Build history of the part. All positions in model axes, mm. A direction names the side the tool comes from. Give positions to 0.01 mm unless a question says otherwise; leave off trailing zeros. Loops run counter-clockwise (first coordinate to the right, second up) from the corner with the lowest first, then second, coordinate; pieces in that order, holes last. Notation, with made-up numbers: (30, 53.5) -> (86, 53.5) arc R6 cw to (86, 63.5) -> close; hole circle Ø1 at (-28, 38). An arc over 180 degrees is marked (long way). One line per question, with ' | ' between items. Start each with the question number.
(1) Mould opens along X. For faces 1 (the face through (-48.22, 2.5, 0.48)), 2 (the face through (11.437, 12.629, -13.635)), 3 (the face through (-0.64, 2.5, 36.79)) say: pulls with the +X half, pulls with the -X half, needs draft (parallel to the pull), parting line crosses it, or undercut.
(2) Slice it at C-C, the plane y = 9. Write the cut outline in (x, z).
(3) Flat gauge pins, fed straight in: pin 1 Ø2 at (x, z) = (30, -6.5) entering from -Y; pin 2 Ø7.5 at (x, z) = (-20, 12.5) entering from -Y; pin 3 Ø17.5 at (y, z) = (41.91, 0) entering from -X. Where does each tip first touch, or does it go through?
(4) Slice it at B-B, the plane x = 4.5. Write the cut outline in (y, z).
(5) 3-axis set-ups, long thin cutter, end or side, ignore diameter. For faces 4 (the face through (48.224, 84.364, -0.373)), 5 (the face through (-1, 7.62, 0)): which of +Z, -Z, +X, -X, +Y, -Y reach the whole face in a straight line?
(6) Drill centre lines: L1, parallel to Z at x = 19, y = 10; L2, parallel to X at y = 12, z = -14.5; L3, parallel to Z at x = 40, y = 41.91. Where is each one in solid material? Low to high. Write a range as from..to.
(7) Slice it at A-A, the plane z = -13.97. Write the cut outline in (x, y), then the cut area to 3 significant figures.
(8) Slice it at D-D, the plane y = 70.5. Write the cut outline in (x, z), then the cut area to 3 significant figures.
```python
from build123d import *

# Parameters (mm, degrees)
F1_DEPTH = 50.8
F2_W     = 76.2
F2_H     = 53.34
F3_DEPTH = 7.62
F4_R     = 7.62
F5_DEPTH = 10.16
F6_R     = 7.62
F7_DEPTH = 19.05
F8_R     = 7.62
F9_DEPTH = 19.05
F10_SIZE = 5.08


with BuildPart() as f1:
    # F0 (on Right) → F1 (new body, symmetric)
    with BuildSketch(Plane.YZ):
        Polygon((41.91, 39.37), (0, 39.37), (0, 0), (0, -39.37), (41.91, -39.37), (86.868, -26.67), (86.868, 0), (86.868, 26.67), align=None)
    extrude(amount=F1_DEPTH, both=True)

    # F2 (on face) → F3 (cut)
    with BuildSketch(Plane.XZ):
        Rectangle(F2_W, F2_H)
    extrude(amount=-F3_DEPTH, mode=Mode.SUBTRACT)

    # F4 (on face) → F5 (cut)
    with BuildSketch(Plane.XZ.offset(-7.62)):
        with Locations((-19.05, 13.97)):
            Circle(F4_R)
        with Locations((19.05, 13.97)):
            Circle(F4_R)
        with Locations((-19.05, -13.97)):
            Circle(F4_R)
        with Locations((19.05, -13.97)):
            Circle(F4_R)
    extrude(amount=-F5_DEPTH, mode=Mode.SUBTRACT)

    # F6 (on face) → F7 (cut)
    with BuildSketch(Plane.YZ.offset(50.8)):
        with Locations((41.91, 0)):
            Circle(F6_R)
    extrude(amount=-F7_DEPTH, mode=Mode.SUBTRACT)

    # F8 (on face) → F9 (cut)
    with BuildSketch(Plane(origin=(-50.8, 0, 0), x_dir=(0, -1, 0), z_dir=(-1, 0, 0))):
        with Locations((-41.91, 0)):
            Circle(F8_R)
    extrude(amount=-F9_DEPTH, mode=Mode.SUBTRACT)

    # F10
    f10_edges = [f1.edges().sort_by_distance(p)[0] for p in [
        (50.8, 20.955, 39.37),
        (50.8, 64.389, 33.02),
        (50.8, 0, 0),
        (50.8, 86.868, 0),
        (50.8, 20.955, -39.37),
        (50.8, 64.389, -33.02),
        (50.8, 34.29, 0),
        (-50.8, 20.955, 39.37),
        (-50.8, 64.389, 33.02),
        (-50.8, 0, 0),
        (-50.8, 86.868, 0),
        (-50.8, 20.955, -39.37),
        (-50.8, 64.389, -33.02),
        (-50.8, 49.53, 0),
        (0, 0, 39.37),
        (0, 0, -39.37),
    ]]
    chamfer(f10_edges, length=F10_SIZE)


solid = f1.part
```
Final values:
1) face 1: pulls with the -X half | face 2: undercut | face 3: needs draft
2) outline: (-50.8, -34.29) -> (-45.72, -39.37) -> (45.72, -39.37) -> (50.8, -34.29) -> (50.8, 34.29) -> (45.72, 39.37) -> (-45.72, 39.37) -> (-50.8, 34.29) -> close; hole circle Ø15.24 at (-19.05, -13.97); hole circle Ø15.24 at (-19.05, 13.97); hole circle Ø15.24 at (19.05, -13.97); hole circle Ø15.24 at (19.05, 13.97)
3) pin 1: y = 7.62 | pin 2: y = 17.78 | pin 3: x = -46.85
4) outline: (0, -34.29) -> (5.08, -39.37) -> (41.91, -39.37) -> (86.87, -26.67) -> (86.87, 26.67) -> (41.91, 39.37) -> (5.08, 39.37) -> (0, 34.29) -> (0, 26.67) -> (7.62, 26.67) -> (7.62, -26.67) -> (0, -26.67) -> close
5) face 4: +Z, -Z, +X, +Y | face 5: -Y
6) L1: -39.37..-21.59, -6.35..6.35, 21.59..39.37 | L2: -50.8..-26.65, -11.45..11.45, 26.65..50.8 | L3: -39.37..-7.62, 7.62..39.37
7) outline: (-50.8, 5.08) -> (-45.72, 0) -> (-38.1, 0) -> (-38.1, 7.62) -> (-26.67, 7.62) -> (-26.67, 17.78) -> (-11.43, 17.78) -> (-11.43, 7.62) -> (11.43, 7.62) -> (11.43, 17.78) -> (26.67, 17.78) -> (26.67, 7.62) -> (38.1, 7.62) -> (38.1, 0) -> (45.72, 0) -> (50.8, 5.08) -> (50.8, 81.79) -> (45.72, 86.87) -> (-45.72, 86.87) -> (-50.8, 81.79) -> close | area: 7,880 mm2
8) outline: (-50.8, -26.01) -> (-45.72, -31.29) -> (45.72, -31.29) -> (50.8, -26.01) -> (50.8, 26.01) -> (45.72, 31.29) -> (-45.72, 31.29) -> (-50.8, 26.01) -> close | area: 6,310 mm2
